from build123d import *

# Parameters (mm, degrees)
SKETCH2_R               = 12.2
BOSS_EXTRUDE1_DEPTH     = 31
FILLET1_R               = 1
SKETCH3_R               = 12.5
BOSS_EXTRUDE2_DEPTH     = 21
SKETCH4_R               = 3.5
BOSS_EXTRUDE3_DEPTH     = 4
SKETCH5_R               = 2
BOSS_EXTRUDE4_DEPTH     = 8
BOSS_EXTRUDE5_START     = 10
SKETCH6_R               = 12.2
BOSS_EXTRUDE5_DEPTH     = 10
CUT_EXTRUDE1_DEPTH      = 20
CUT_EXTRUDE1_DEPTH_BACK = 19
SKETCH7_W               = 2.212937173
SKETCH7_H               = 31.307930015


with BuildPart() as part:
    # Sketch2 → Boss-Extrude1 (new body)
    with BuildSketch(Plane.XY):
        Circle(SKETCH2_R)
    extrude(amount=BOSS_EXTRUDE1_DEPTH)

    # Fillet1
    fillet1_edges = [part.edges().sort_by_distance(p)[0] for p in [
        (-12.2, 0, 31),
    ]]
    fillet(fillet1_edges, radius=FILLET1_R)

    # Sketch3 → Boss-Extrude2 (add)
    with BuildSketch(Plane.XY.offset(31)):
        with Locations(Location((0, 0, 0), (0, 0, 180))):
            Circle(SKETCH3_R)
    extrude(amount=BOSS_EXTRUDE2_DEPTH)

    # Sketch4 → Boss-Extrude3 (add)
    with BuildSketch(Plane.XY.offset(52)):
        Circle(SKETCH4_R)
    extrude(amount=BOSS_EXTRUDE3_DEPTH)

    # Sketch5 → Boss-Extrude4 (add)
    with BuildSketch(Plane.XY.offset(56)):
        Circle(SKETCH5_R)
    extrude(amount=BOSS_EXTRUDE4_DEPTH)

    # Sketch6 → Boss-Extrude5 (add)
    with BuildSketch(Plane(origin=(0, 0, 0), x_dir=(-1, 0, 0), z_dir=(0, 0, -1)).offset(BOSS_EXTRUDE5_START)):
        Circle(SKETCH6_R)
    extrude(amount=-BOSS_EXTRUDE5_DEPTH)

    # Sketch7 → Cut-Extrude1 (cut, two sides: drawn at the far end of the back side and taken through both)
    with BuildSketch(Plane(origin=(0, 0, 0), x_dir=(0, 0, -1), z_dir=(1, 0, 0)).offset(-CUT_EXTRUDE1_DEPTH_BACK)):
        with Locations((10.106468587, 3.153965008)):
            Rectangle(SKETCH7_W, SKETCH7_H)
    extrude(amount=CUT_EXTRUDE1_DEPTH + CUT_EXTRUDE1_DEPTH_BACK, mode=Mode.SUBTRACT)


solid = part.part
Read the model definition and answer for the solid it produces. Units are mm, in the model's axes. A direction names the side the tool comes from. Coordinates: 2 decimals unless noted, no trailing zeros. Write each loop counter-clockwise with the first axis right and the second up, starting at its lowest first coordinate (ties: lowest second). Pieces come first, ordered by that corner, then holes. Notation, with made-up numbers: M 51,-38 L 60,-38 A26 ccw 60,-23 Z; hole C 37.25,42 d4. An arc over 180 degrees is marked long. Use a Markdown table: item, result.
Q1. Straight lines are drawn through the part: L1, parallel to Z at x = 5.5, y = -3; L2, parallel to Y at x = -0.5, z = 9.5; L3, parallel to Z at x = 11.5, y = -4.75. For each, find the intervals that lie inside material, in ascending order. Write a range as [from, to].
Answer block:
| item | result |
|---|---|
| L1 | z = [-9, 52] |
| L2 | y = [-12.19, 12.19] |
| L3 | z = [31, 52] |
Q2. The part is cut by section D-D, the plane z = 51. Write down the section's boundary in (x, y), then the cut area to 3 significant figures.
Answer block:
| item | result |
|---|---|
| outline | C 0,0 d25 |
| area | 491 mm2 |
Q3. The part is cut by section C-C, the plane z = 24. Write down the section's boundary in (x, y), then the cut area to 3 significant figures.
Answer block:
| item | result |
|---|---|
| outline | C 0,0 d24.4 |
| area | 468 mm2 |
Q4. Each of these flat-tipped pins is pushed along its axis until it touches: pin 1 Ø2 at (x, z) = (-5, 0.5) entering from -Y; pin 2 Ø6 at (x, z) = (-6, 40.5) entering from -Y; pin 3 Ø1.5 at (x, z) = (3.5, 37.5) entering from +Y. Where does it stop, or does it pass through?
Answer block:
| item | result |
|---|---|
| pin 1 | stops at y = -11.53 |
| pin 2 | stops at y = -12.13 |
| pin 3 | stops at y = 12.19 |
Q5. The part is cut by section A-A, the plane y = 0. Write down the section's boundary in (x, z).
Answer block:
| item | result |
|---|---|
| outline | M -12.5,31 L -11.2,31 A1 ccw -12.2,30 L -12.2,-9 L 12.2,-9 L 12.2,30 A1 ccw 11.2,31 L 12.5,31 L 12.5,52 L 3.5,52 L 3.5,56 L 2,56 L 2,64 L -2,64 L -2,56 L -3.5,56 L -3.5,52 L -12.5,52 Z |
Q6. Which of the six approach directions +Z, -Z, +X, -X, +Y, -Y give full straight-line access (tool end or side, diameter ignored) to faces 1 (the face through (0, -2, 60)), 2 (the face through (0, 0, 64))?
Answer block:
| item | result |
|---|---|
| face 1 | +Z |
| face 2 | +Z, +X, -X, +Y, -Y |
